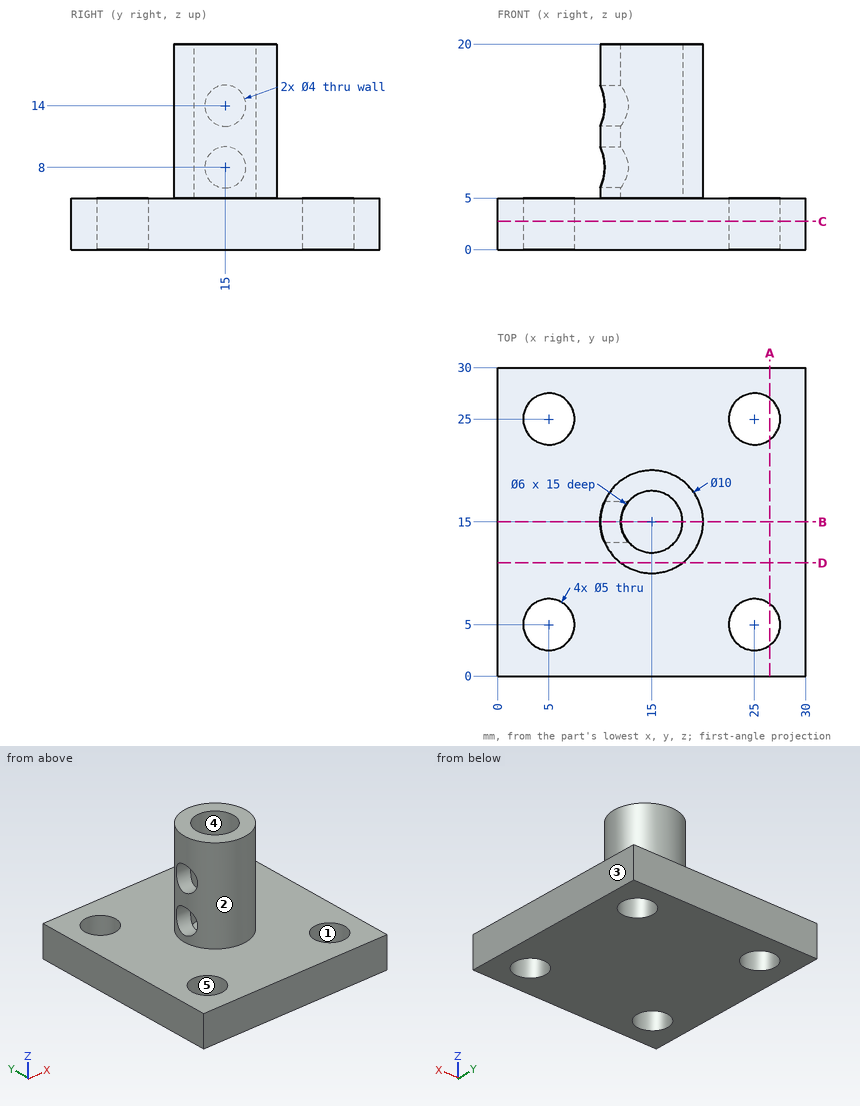
Study the drawing (mm; zero at the part's minimum x, y, z) and answer. A direction names the side the tool comes from. Round coordinates to 2 decimals unless told otherwise and drop trailing zeros. Write each loop counter-clockwise with the first axis right and the second up, starting at its lowest first coordinate (ties: lowest second). Pieces come first, ordered by that corner, then holes. Notation, with made-up numbers: (-11, -31.75) -> (26, -31.75) arc R9 cw to (26, -15.75) -> close; hole circle Ø9 at (-2.75, 71). An arc over 180 degrees is marked (long way). Use CSV: the item, a comma, the result in double quotes. Start each with the question number.
(1) Consider L1, parallel to Y at x = 5, z = 3.1; L2, parallel to Y at x = 15, z = 16.75; L3, parallel to Y at x = 25.75, z = 3. Determine where each line is inside the solid, lowest interval first. Write a range as from..to.
(2) Section A-A on x = 26.5 is taken. Give the vertices of the cut face in (y, z), then the cut area to 3 significant figures.
(3) Section C-C on z = 2.75 is taken. Give the vertices of the cut face in (x, y).
(4) Section B-B on y = 15 is taken. Give the vertices of the cut face in (x, z), then the cut area to 3 significant figures.
(5) The mould has two halves that part along X. Classify the marked faces 1, 2 and 3: released by +X, released by -X, zero draft, split by the parting line, or undercut.
(6) Section D-D on y = 11 is taken. Give the vertices of the cut face in (x, z).
(7) Which of the six approach directions +Z, -Z, +X, -X, +Y, -Y give full straight-line access (tool end or side, diameter ignored) to the marked faces 4 and 5?
(8) Each of these flat-tipped pins is pushed along its axis until it touches: pin 1 (6 mm diameter, centred on x = 25, y = 25, fed in from -Z); pin 2 (2 mm diameter, centred on x = 11.5, z = 7, fed in from -Y); pin 3 (1 mm diameter, centred on x = 3, z = 6, fed in from -Y); pin 4 (1 mm diameter, centred on y = 17, z = 14.5, fed in from +X). Where does it stop, or does it pass through?
A:
1,L1,"y = 0..2.5, 7.5..22.5, 27.5..30"
1,L2,"y = 10..12, 18..20"
1,L3,"y = 0..2.62, 7.38..22.62, 27.38..30"
2,outline,"(0, 0) -> (3, 0) -> (3, 5) -> (0, 5) -> close; (7, 0) -> (23, 0) -> (23, 5) -> (7, 5) -> close; (27, 0) -> (30, 0) -> (30, 5) -> (27, 5) -> close"
2,area,"110 mm²"
3,outline,"(0, 0) -> (30, 0) -> (30, 30) -> (0, 30) -> close; hole circle Ø5 at (5, 5); hole circle Ø5 at (5, 25); hole circle Ø5 at (25, 5); hole circle Ø5 at (25, 25)"
4,outline,"(0, 0) -> (30, 0) -> (30, 5) -> (20, 5) -> (20, 20) -> (18, 20) -> (18, 5) -> (12, 5) -> (12, 6) -> (10, 6) -> (10, 5) -> (0, 5) -> close; (10, 10) -> (12, 10) -> (12, 12) -> (10, 12) -> close; (10, 16) -> (12, 16) -> (12, 20) -> (10, 20) -> close"
4,area,"194 mm²"
5,face 1,"undercut"
5,face 2,"split by the parting line"
5,face 3,"released by +X"
6,outline,"(0, 0) -> (30, 0) -> (30, 5) -> (18, 5) -> (18, 20) -> (12, 20) -> (12, 5) -> (0, 5) -> close"
7,face 4,"+Z"
7,face 5,"+Z, -Z"
8,pin 1,"stops at z = 0"
8,pin 2,"stops at y = 10.67"
8,pin 3,"passes through"
8,pin 4,"stops at x = 19.77"
